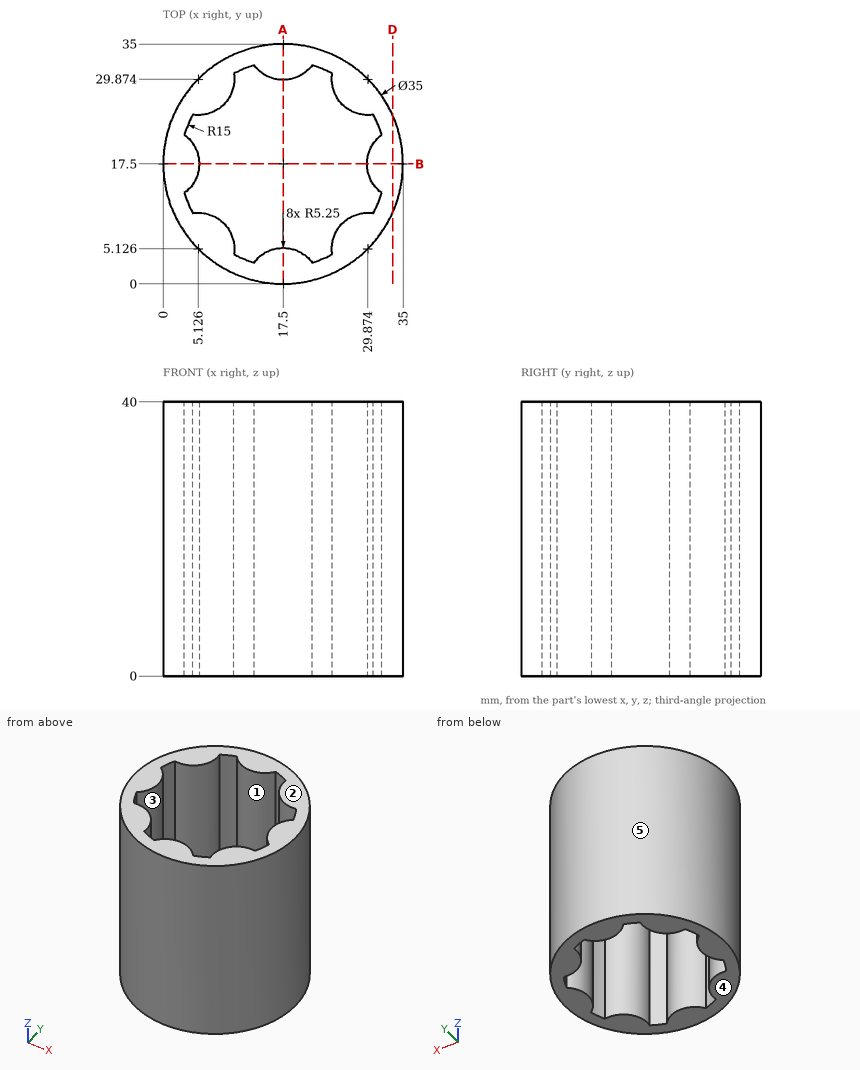
Check sheet for the drawn part. Datum: minimum x, y, z corner. Units: mm. A direction names the side the tool comes from. Give positions to 0.01 mm unless a question says otherwise; leave off trailing zeros. Write each loop counter-clockwise with the first axis right and the second up, starting at its lowest first coordinate (ties: lowest second). Pieces come first, ordered by that corner, then holes. Notation, with made-up numbers: M 28,74 L 87,74 A35 cw 87,108 Z; hole C 54,63 d9. An arc over 180 degrees is marked long. Write item = value, one per line.
(1) Sectioned sample at A-A (x = 17.5). Record the cut outline in (y, z), then the cut area to 3 significant figures.
Found:
outline = M 0,0 L 5.25,0 L 5.25,40 L 0,40 Z; M 29.75,0 L 35,0 L 35,40 L 29.75,40 Z
area = 420 mm2
(2) Draft check along X on the marked faces 3, 4 and 5. Enter one of: released by +X, released by -X, zero draft, split by the parting line, or undercut.
Found:
face_3 = undercut
face_4 = zero draft
face_5 = split by the parting line
(3) Access from +Z, -Z, +X, -X, +Y, -Y to the whole of each face (thin tool, end or side, straight path). Record for the marked faces 1 and 2.
Found:
face_1 = +Z, -Z
face_2 = +Z, +X, -X, +Y, -Y
(4) Go/stop test with flat-tipped pins: pin 1 Ø5 at (x, z) = (22, 33) entering from -Y (1 decimal); pin 2 Ø3 at (y, z) = (7.5, 16) entering from -X; pin 3 Ø10 at (x, y) = (17.5, 14.5) entering from -Z; pin 4 Ø12 at (y, z) = (24.5, 14.5) entering from -X. Record where each tip stops, or that it passes through.
Found:
pin_1 = 0.1
pin_2 = 2.2
pin_3 = through
pin_4 = 0.03
(5) Material ranges on line 1 (X direction, y = 31, z = 15.5) (1 decimal); line 2 (X direction, y = 23.5, z = 15.5), recorded low to high.
Found:
line_1 = 6.4 to 11, 14.1 to 20.9, 24 to 28.6
line_2 = 1.06 to 3.75, 31.25 to 33.94
(6) Sectioned sample at D-D (x = 33.5). Record the cut outline in (y, z), then the cut area to 3 significant figures.
Found:
outline = M 10.41,0 L 24.59,0 L 24.59,40 L 10.41,40 Z
area = 567 mm2
